Source: CAD feature listing. Evaluate the final solid. Frame: model axes, mm. A direction names the side the tool comes from. Round coordinates to 2 decimals unless told otherwise and drop trailing zeros. Write each loop counter-clockwise with the first axis right and the second up, starting at its lowest first coordinate (ties: lowest second). Pieces come first, ordered by that corner, then holes.
from build123d import *

# Parameters (mm, degrees)
SKETCH_2_W               = 27
SKETCH_2_H               = 10
EXTRUDE_1_DEPTH          = 17.5
SKETCH_4_R               = 1.5
CUT_EXTRUDE_1_DEPTH      = 4
SKETCH_6_W               = 27
SKETCH_6_H               = 0.5
CUT_EXTRUDE_2_DEPTH      = 0.5
SKETCH_7_W               = 0.5
SKETCH_7_H               = 9.5
CUT_EXTRUDE_3_DEPTH      = 0.5
SKETCH_12_W              = 27
SKETCH_12_H              = 10
SKETCH_12_W_2            = 26.8
SKETCH_12_H_2            = 9.8
CUT_EXTRUDE_5_DEPTH      = 2
MIRROR_3_COPY_1_SKETCH_W = 0.5
MIRROR_3_COPY_1_SKETCH_H = 9.5
MIRROR_3_COPY_1_DEPTH    = 0.5
MIRROR_3_COPY_2_SKETCH_W = 27
MIRROR_3_COPY_2_SKETCH_H = 0.5
MIRROR_3_COPY_2_DEPTH    = 0.5
SKETCH_5_W               = 13
SKETCH_5_H               = 9.581228834
CUT_EXTRUDE_4_DEPTH      = 97
EXTRUDE_3_DEPTH          = 35


with BuildPart() as part:
    # 草图2 → 凸台-拉伸1 (new body, symmetric)
    with BuildSketch(Plane.XY):
        Rectangle(SKETCH_2_W, SKETCH_2_H)
    extrude(amount=EXTRUDE_1_DEPTH, both=True)

    # 草图4 → 切除-拉伸1 (cut)
    with BuildSketch(Plane(origin=(0, 5, 0), x_dir=(1, 0, 0), z_dir=(0, 1, 0))):
        with Locations((-10, 7.5)):
            Circle(SKETCH_4_R)
        with Locations((10, 7.5)):
            Circle(SKETCH_4_R)
        with Locations((-10, -7.5)):
            Circle(SKETCH_4_R)
        with Locations((10, -7.5)):
            Circle(SKETCH_4_R)
    extrude(amount=-CUT_EXTRUDE_1_DEPTH, mode=Mode.SUBTRACT)

    # 草图6 → 切除-拉伸2 (cut)
    with BuildSketch(Plane(origin=(0, 5, 0), x_dir=(1, 0, 0), z_dir=(0, 1, 0))):
        with Locations((0, 10)):
            Rectangle(SKETCH_6_W, SKETCH_6_H)
    cut_extrude_2 = extrude(amount=-CUT_EXTRUDE_2_DEPTH, mode=Mode.SUBTRACT)

    # 草图7 → 切除-拉伸3 (cut)
    with BuildSketch(Plane.ZY.offset(13.5)):
        with Locations((-10, -0.25)):
            Rectangle(SKETCH_7_W, SKETCH_7_H)
    cut_extrude_3 = extrude(amount=-CUT_EXTRUDE_3_DEPTH, mode=Mode.SUBTRACT)

    # 草图12 → 切除-拉伸5 (cut)
    with BuildSketch(Plane(origin=(0, 0, -17.5), x_dir=(-1, 0, 0), z_dir=(0, 0, -1))):
        Rectangle(SKETCH_12_W, SKETCH_12_H)
        Rectangle(SKETCH_12_W_2, SKETCH_12_H_2, mode=Mode.SUBTRACT)
    cut_extrude_5 = extrude(amount=-CUT_EXTRUDE_5_DEPTH, mode=Mode.SUBTRACT)

    # 镜向1: 切除-拉伸2 across plane
    add(cut_extrude_2.mirror(Plane.ZX), mode=Mode.SUBTRACT)

    # 镜向2: 切除-拉伸3 across plane
    add(cut_extrude_3.mirror(Plane(origin=(0, 0, 0), x_dir=(0, 0, 1), z_dir=(1, 0, 0))), mode=Mode.SUBTRACT)

    # 镜向3: 切除-拉伸5, 切除-拉伸2, 切除-拉伸3 across plane
    add(cut_extrude_5.mirror(Plane.XY), mode=Mode.SUBTRACT)
    add(cut_extrude_2.mirror(Plane.XY), mode=Mode.SUBTRACT)
    add(cut_extrude_3.mirror(Plane.XY), mode=Mode.SUBTRACT)

    # 镜向3 copy 1 sketch → 镜向3 copy 1 (cut)
    with BuildSketch(Plane(origin=(13.5, 0, 0), x_dir=(0, 0, -1), z_dir=(1, 0, 0))):
        with Locations((-10, -0.25)):
            Rectangle(MIRROR_3_COPY_1_SKETCH_W, MIRROR_3_COPY_1_SKETCH_H)
    extrude(amount=-MIRROR_3_COPY_1_DEPTH, mode=Mode.SUBTRACT)

    # 镜向3 copy 2 sketch → 镜向3 copy 2 (cut)
    with BuildSketch(Plane.XZ.offset(5)):
        with Locations((0, 10)):
            Rectangle(MIRROR_3_COPY_2_SKETCH_W, MIRROR_3_COPY_2_SKETCH_H)
    extrude(amount=-MIRROR_3_COPY_2_DEPTH, mode=Mode.SUBTRACT)

    # 草图5 → 切除-拉伸4 (cut)
    with BuildSketch(Plane.XY.offset(17.5)):
        with Locations((0, -4.290614417)):
            Rectangle(SKETCH_5_W, SKETCH_5_H)
    extrude(amount=-CUT_EXTRUDE_4_DEPTH, mode=Mode.SUBTRACT)

    # 草图9 → 凸台-拉伸3 (add)
    with BuildSketch(Plane.XY.offset(17.5)):
        Polygon((-6.5, -1.1), (-5.5, -1.6), (-5.5, -2.4), (-6.5, -2.9), align=None)
        Polygon((5.5, -1.6), (5.5, -2.4), (6.5, -2.9), (6.5, -1.1), align=None)
    extrude(amount=-EXTRUDE_3_DEPTH)


solid = part.part
1) Reachability of faces 4 (the face through (-10, -4.9, 17)), 5 (the face through (0, 0.5, 0)), 6 (the face through (-6.5, -4, 0)), 7 (the face through (10, 3, -6)), 8 (the face through (13.4, 0, 17)) from +Z, -Z, +X, -X, +Y, -Y: full face, straight path, thin tool, end or side. Return the list, or none.
Taken from the geometry:
face 4: +Z, +X, -X, -Y
face 5: +Z, -Z
face 6: +Z, -Z, -Y
face 7: +Y
face 8: +Z, +X, +Y, -Y
2) Section query B-B on z = -5. Return the cut outline in (x, y), then the cut area to 3 significant figures.
Taken from the geometry:
outline: (-13.5, -5) - (-6.5, -5) - (-6.5, -2.9) - (-5.5, -2.4) - (-5.5, -1.6) - (-6.5, -1.1) - (-6.5, 0.5) - (6.5, 0.5) - (6.5, -1.1) - (5.5, -1.6) - (5.5, -2.4) - (6.5, -2.9) - (6.5, -5) - (13.5, -5) - (13.5, 5) - (-13.5, 5) - close
area: 201 mm2
3) Section query C-C on y = 1.75. State how many separate pieces and enclosed holes the cut face has, then the cut area to 3 significant figures.
Taken from the geometry:
separate pieces: 1
enclosed holes: 4
area: 915 mm2
4) Pull-direction query (Z, two-part tool) for faces 1 (the face through (0, 1, -17.5)), 2 (the face through (0, 5, -13)), 3 (the face through (-5.1, 4.8, -10.25)); classes: released by +Z, released by -Z, zero draft, split by the parting line, or undercut.
Taken from the geometry:
face 1: released by -Z
face 2: zero draft
face 3: undercut
5) Contact query for flat-ended pins moving along their axis: P1, Ø0.6, axis at y = 0, z = 16.5, coming from the +X side; P2, Ø1.5, axis at x = -9.5, z = 7, coming from the +Y side; P3, Ø2, axis at x = 9.5, z = -17, coming from the -Y side. Output: stop coordinate, or through.
Taken from the geometry:
P1: stops at x = 13.4
P2: stops at y = 1
P3: stops at y = -4.9
6) Material intervals for line 1 (X direction, y = 3.7, z = -7.5); line 2 (Z direction, x = 10, y = 3.2); line 3 (X direction, y = -1, z = 6), sorted ascending.
Taken from the geometry:
line 1: x = -13.5 to -11.5, -8.5 to 8.5, 11.5 to 13.5
line 2: z = -17.5 to -9, -6 to 6, 9 to 17.5
line 3: x = -13.5 to -6.5, 6.5 to 13.5
